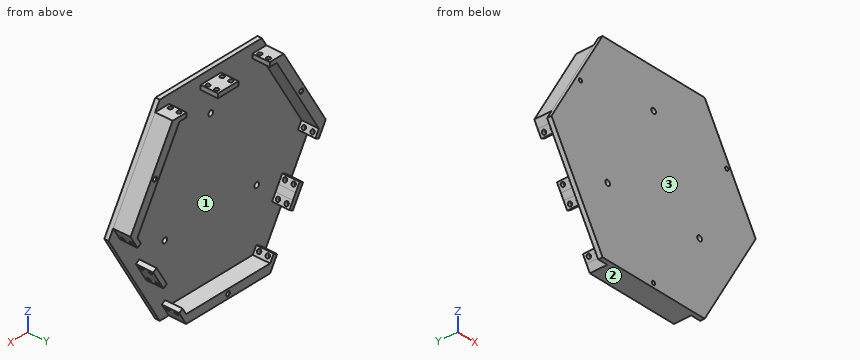
from build123d import *

# Parameters (mm, degrees)
EXTRUDE_5_DEPTH              = 5
SKETCH_7_W                   = 9
SKETCH_7_H                   = 5
SKETCH_7_W_2                 = 8
EXTRUDE_6_DEPTH              = 20
EXTRUDE_7_DEPTH              = 20
SKETCH_13_R                  = 2.3
CUT_EXTRUDE_2_DEPTH          = 20
SKETCH_9_R                   = 2.3
CUT_EXTRUDE_3_DEPTH          = 20
SKETCH_11_R                  = 2.3
CUT_EXTRUDE_4_DEPTH          = 20
SKETCH_16_R                  = 3
CUT_EXTRUDE_5_DEPTH          = 5
HOLE_WIZARD_M5_1_D           = 4.2
HOLE_WIZARD_M5_1_CSINK_D     = 5.05
HOLE_WIZARD_M5_1_CSINK_ANGLE = 90


with BuildPart() as part:
    # 草图6 → 凸台-拉伸5 (new body)
    with BuildSketch(Plane(origin=(0, 0, 0), x_dir=(1, 0, 0), z_dir=(0, 1, 0))):
        Polygon((130, 0), (65, 112.583302492), (-65, 112.583302492), (-130, 0), (-65, -112.583302492), (65, -112.583302492), align=None)
    extrude(amount=EXTRUDE_5_DEPTH)

    # 草图7 → 凸台-拉伸6 (add)
    with BuildSketch(Plane(origin=(0, 5, 0), x_dir=(1, 0, 0), z_dir=(0, 1, 0))):
        with Locations((57.5, -100.083302492)):
            Rectangle(SKETCH_7_W, SKETCH_7_H)
        with Locations((8.5, -100.083302492)):
            Rectangle(SKETCH_7_W, SKETCH_7_H)
        with Locations((0, -100.083302492)):
            Rectangle(SKETCH_7_W_2, SKETCH_7_H)
        with Locations((-8.5, -100.083302492)):
            Rectangle(SKETCH_7_W, SKETCH_7_H)
        with Locations((-57.5, -100.083302492)):
            Rectangle(SKETCH_7_W, SKETCH_7_H)
        Polygon((115.339745962, 5.392304845), (119.839745962, -2.401923789), (115.509618943, -4.901923789), (111.009618943, 2.892304845), align=None)
        Polygon((95.339745962, 40.033320997), (91.009618943, 37.533320997), (86.009618943, 46.193575035), (90.339745962, 48.693575035), align=None)
        Polygon((86.839745962, 54.755752861), (82.509618943, 52.255752861), (86.009618943, 46.193575035), (90.339745962, 48.693575035), align=None)
        Polygon((82.339745962, 62.549981495), (86.839745962, 54.755752861), (82.509618943, 52.255752861), (78.009618943, 60.049981495), align=None)
        Polygon((62.339745962, 97.190997647), (58.009618943, 94.690997647), (53.509618943, 102.485226281), (57.839745962, 104.985226281), align=None)
        Polygon((-57.839745962, 104.985226281), (-53.509618943, 102.485226281), (-58.009618943, 94.690997647), (-62.339745962, 97.190997647), align=None)
        Polygon((-82.339745962, 62.549981495), (-86.839745962, 54.755752861), (-82.509618943, 52.255752861), (-78.009618943, 60.049981495), align=None)
        Polygon((-86.839745962, 54.755752861), (-82.509618943, 52.255752861), (-86.009618943, 46.193575035), (-90.339745962, 48.693575035), align=None)
        Polygon((-90.339745962, 48.693575035), (-86.009618943, 46.193575035), (-91.009618943, 37.533320997), (-95.339745962, 40.033320997), align=None)
        Polygon((-115.339745962, 5.392304845), (-119.839745962, -2.401923789), (-115.509618943, -4.901923789), (-111.009618943, 2.892304845), align=None)
    extrude(amount=EXTRUDE_6_DEPTH)

    # 草图10 → 凸台-拉伸7 (add)
    with BuildSketch(Plane(origin=(0, 5, 0), x_dir=(1, 0, 0), z_dir=(0, 1, 0))):
        Polygon((-115.509618943, -4.901923789), (-62, -97.583302492), (-62, -102.583302492), (-70.773502692, -102.583302492), (-124.226497308, -10), (-119.839745962, -2.401923789), align=None)
        Polygon((62, -97.583302492), (115.509618943, -4.901923789), (119.839745962, -2.401923789), (124.226497308, -10), (70.773502692, -102.583302492), (62, -102.583302492), align=None)
        Polygon((57.839745962, 104.985226281), (53.509618943, 102.485226281), (-53.509618943, 102.485226281), (-57.839745962, 104.985226281), (-53.509618943, 112.583302492), (53.452994616, 112.583302492), align=None)
    extrude(amount=EXTRUDE_7_DEPTH)

    # 草图13 → 切除-拉伸2 (cut)
    with BuildSketch(Plane(origin=(-88.839745962, 0, -51.291651246), x_dir=(-0.5000000000000006, 0, 0.8660254037844384), z_dir=(-0.8660254037844384, 0, -0.5000000000000006))):
        with Locations((-57, 20)):
            Circle(SKETCH_13_R)
        with Locations((-57, 10)):
            Circle(SKETCH_13_R)
        with Locations((-9, 20)):
            Circle(SKETCH_13_R)
        with Locations((-9, 10)):
            Circle(SKETCH_13_R)
        with Locations(Location((9, 10, 0), (0, 0, 180))):
            Circle(SKETCH_13_R)
        with Locations(Location((9, 20, 0), (0, 0, 180))):
            Circle(SKETCH_13_R)
        with Locations(Location((57, 10, 0), (0, 0, 180))):
            Circle(SKETCH_13_R)
        with Locations(Location((57, 20, 0), (0, 0, 180))):
            Circle(SKETCH_13_R)
    extrude(amount=-CUT_EXTRUDE_2_DEPTH, mode=Mode.SUBTRACT)

    # 草图9 → 切除-拉伸3 (cut)
    with BuildSketch(Plane.XY.offset(102.583302492)):
        with Locations((-57, 20)):
            Circle(SKETCH_9_R)
        with Locations((-57, 10)):
            Circle(SKETCH_9_R)
        with Locations((-9, 20)):
            Circle(SKETCH_9_R)
        with Locations((-9, 10)):
            Circle(SKETCH_9_R)
        with Locations((9, 20)):
            Circle(SKETCH_9_R)
        with Locations((9, 10)):
            Circle(SKETCH_9_R)
        with Locations((57, 20)):
            Circle(SKETCH_9_R)
        with Locations((57, 10)):
            Circle(SKETCH_9_R)
    extrude(amount=-CUT_EXTRUDE_3_DEPTH, mode=Mode.SUBTRACT)

    # 草图11 → 切除-拉伸4 (cut)
    with BuildSketch(Plane(origin=(88.839745962, 0, -51.291651246), x_dir=(-0.5000000000000029, 0, -0.866025403784437), z_dir=(0.8660254037844369, 0, -0.5000000000000028))):
        with Locations((-57, 20)):
            Circle(SKETCH_11_R)
        with Locations((-57, 9.847641324)):
            Circle(SKETCH_11_R)
        with Locations((-9, 20)):
            Circle(SKETCH_11_R)
        with Locations((-9, 9.847641324)):
            Circle(SKETCH_11_R)
        with Locations(Location((9, 9.847641324, 0), (0, 0, 180))):
            Circle(SKETCH_11_R)
        with Locations(Location((9, 20, 0), (0, 0, 180))):
            Circle(SKETCH_11_R)
        with Locations(Location((57, 9.847641324, 0), (0, 0, 180))):
            Circle(SKETCH_11_R)
        with Locations(Location((57, 20, 0), (0, 0, 180))):
            Circle(SKETCH_11_R)
    extrude(amount=-CUT_EXTRUDE_4_DEPTH, mode=Mode.SUBTRACT)

    # 草图16 → 切除-拉伸5 (cut)
    with BuildSketch(Plane(origin=(0, 5, 0), x_dir=(1, 0, 0), z_dir=(0, 1, 0))):
        with Locations(Location((0, -67.583302492, 0), (0, 0, 270))):
            Circle(SKETCH_16_R)
        with Locations(Location((58.52885683, 33.791651246, 0), (0, 0, 270))):
            Circle(SKETCH_16_R)
        with Locations(Location((-58.52885683, 33.791651246, 0), (0, 0, 270))):
            Circle(SKETCH_16_R)
    extrude(amount=-CUT_EXTRUDE_5_DEPTH, mode=Mode.SUBTRACT)

    # M5 螺纹孔1 (through all)
    with Locations(Plane(origin=(0, 25, 0), x_dir=(1, 0, 0), z_dir=(0, 1, 0))):
        with Locations((93.127404736, -53.767132193), (-93.127404736, -53.767132193), (-0.014156082, 107.534264386)):
            CounterSinkHole(HOLE_WIZARD_M5_1_D / 2, HOLE_WIZARD_M5_1_CSINK_D / 2, counter_sink_angle=HOLE_WIZARD_M5_1_CSINK_ANGLE)


solid = part.part
Check sheet for the modelled part. Datum: model origin and axes. Units: mm. Face numbers are marked on the shaded views. Round coordinates to 2 decimals unless told otherwise and drop trailing zeros. Write each loop counter-clockwise with the first axis right and the second up, starting at its lowest first coordinate (ties: lowest second). Pieces come first, ordered by that corner, then holes. Notation, with made-up numbers: (17.5, 39) - (65.5, 39) arc R20 cw to (65.5, 78) - close; hole circle Ø10 at (68, 60). An arc over 180 degrees is marked (long way). Return JSON: item names as keys, results as strings.
Q1. Draft check along Z on the marked faces 1, 2 and 3. Enter one of: released by +Z, released by -Z, zero draft, split by the parting line, or undercut.
Returned:
{"face 1": "undercut", "face 2": "released by -Z", "face 3": "zero draft"}
Q2. Depth check by flat-ended pin: P1, Ø3.5, axis at x = -57, y = 20, coming from the -Z side; P2, Ø5, axis at x = -58.53, z = -33.79, coming from the +Y side; P3, Ø12, axis at x = 42.5, y = 16, coming from the +Z side; P4, Ø14, axis at x = 58.5, y = 18.5, coming from the +Z side. Enter the tip coordinate at first touch or a pass-through.
Returned:
{"P1": "stops at z = -109.53", "P2": "passes through", "P3": "stops at z = -102.49", "P4": "stops at z = 102.58"}
Q3. Scan lines: L1, parallel to Y at x = 57, z = 101; L2, parallel to Z at x = -27, y = 16.25; L3, parallel to Y at x = 55, z = -99.5. Record each from-to range of solid material in increasing order. Write a range as from..to.
Returned:
{"L1": "y = 0..7.7, 12.3..17.7, 22.3..25", "L2": "z = -112.58..-102.49", "L3": "y = 0..5"}
Q4. Cross-section at B-B (z = 32). Record the boundary of the cut face in (x, y), then the cut area to 3 significant figures.
Returned:
{"outline": "(-111.52, 0) - (111.52, 0) - (111.52, 25) - (99.86, 25) - (99.86, 5) - (-99.86, 5) - (-99.86, 25) - (-111.52, 25) - close", "area": "1,580 mm²"}
Q5. Cross-section at A-A (x = -32.5). Record the boundary of the cut face in (y, z), then the cut area to 3 significant figures.
Returned:
{"outline": "(0, -112.58) - (25, -112.58) - (25, -102.49) - (5, -102.49) - (5, 112.58) - (0, 112.58) - close", "area": "1,330 mm²"}
